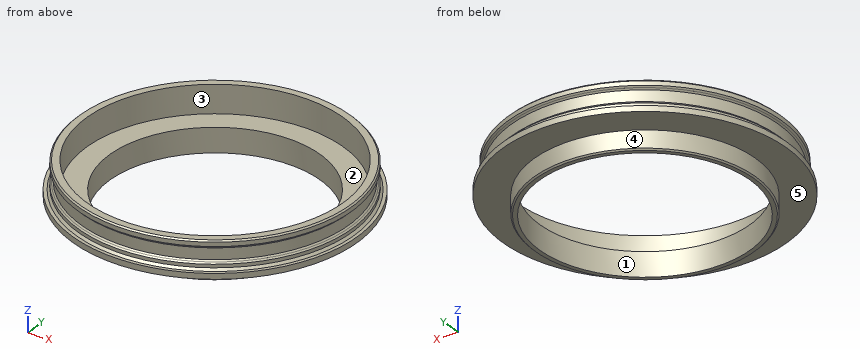
```python
from build123d import *

# Parameters (mm, degrees)
CHAMFER1_SIZE = 0.5
CHAMFER2_SIZE = 0.8


with BuildPart() as part:
    # Sketch1 → Revolve1 (revolve)
    with BuildSketch(Plane(origin=(0, 0, 0), x_dir=(1, 0, 0), z_dir=(0, 1, 0)), mode=Mode.PRIVATE) as revolve1_sk:
        Polygon((37.78, 0), (37.78, -8.7), (46, -8.7), (46, -18.7), (49, -18.7), (49, -16.2), (48, -16.2), (48, -11.2), (49, -11.2), (49, -8.7), (51, -8.7), (51, -6.7), (39.78, -6.7), (39.78, 0), align=None)
    revolve(revolve1_sk.sketch.rotate(Axis((0, 0, -73.981367368), (0, 0, 1)), 180), axis=Axis((0, 0, -73.981367368), (0, 0, 1)))

    # Chamfer1
    chamfer1_edges = [part.edges().sort_by_distance(p)[0] for p in [
        (49, 0, 11.2),
        (48, 0, 11.2),
        (48, 0, 16.2),
        (49, 0, 16.2),
        (49, 0, 18.7),
        (39.78, 0, 0),
    ]]
    chamfer(chamfer1_edges, length=CHAMFER1_SIZE - 0.0001)  # a hair under: the kernel refuses the full size

    # Chamfer2
    chamfer2_edges = [part.edges().sort_by_distance(p)[0] for p in [
        (49, 0, 8.7),
    ]]
    chamfer(chamfer2_edges, length=CHAMFER2_SIZE)


solid = part.part
```
Read the model definition and answer for the solid it produces. Units are mm, in the model's axes. Face numbers are marked on the shaded views. A direction names the side the tool comes from. Coordinates: 2 decimals unless noted, no trailing zeros. Write each loop counter-clockwise with the first axis right and the second up, starting at its lowest first coordinate (ties: lowest second). Pieces come first, ordered by that corner, then holes. Notation, with made-up numbers: (-12, 35.25) -> (37, 35.25) arc R25 cw to (37, 57.25) -> close; hole circle Ø9 at (60.5, 67.25). An arc over 180 degrees is marked (long way). Return JSON: item names as keys, results as strings.
1. Determine the mould class of the marked faces 3, 4 and 5 for opening direction X: pulls with the +X half, pulls with the -X half, needs draft (parallel to the pull), parting line crosses it, or undercut.
Found:
{"face 3": "undercut", "face 4": "parting line crosses it", "face 5": "needs draft"}
2. A tool of negligible diameter and unlimited length cuts with its end or side. For the marked faces 1 and 2, from which of +Z, -Z, +X, -X, +Y, -Y can it reach the whole face along a straight path? Write none if from no direction.
Found:
{"face 1": "+Z, -Z", "face 2": "+Z"}
3. A cutting plane is placed at A-A (z = 4). Determine the outline of the cut face in (x, y), and give its area (3 significant figures).
Found:
{"outline": "circle Ø79.56 at (0, 0); hole circle Ø75.56 at (0, 0)", "area": "487 mm2"}
4. Find the intervals of material crossed by line 1 along Y through (x, z) = (0, 2.5); line 2 along Y through (x, z) = (-17.5, 6.5); line 3 along X through (y, z) = (35, 11.5), in increasing order. Write a range as from..to.
Found:
{"line 1": "-39.78..-37.78, 37.78..39.78", "line 2": "-35.72..-33.48, 33.48..35.72", "line 3": "-33.14..-29.85, 29.85..33.14"}
5. Each of these flat-tipped pins is pushed along its axis until it touches: P1, Ø4, axis at x = 27, z = 3, coming from the -Y side; P2, Ø6, axis at x = 3.5, z = 15, coming from the +Y side; P3, Ø10, axis at x = 29, z = 15.5, coming from the -Y side. Where does it stop, or does it pass through?
Found:
{"P1": "y = -30.94", "P2": "y = 48.99", "P3": "y = -42.64"}
